Check sheet for the modelled part. Datum: model origin and axes. Units: mm. A direction names the side the tool comes from. Give positions to 0.01 mm unless a question says otherwise; leave off trailing zeros. Loops run counter-clockwise (first coordinate to the right, second up) from the corner with the lowest first, then second, coordinate; pieces in that order, holes last. Notation, with made-up numbers: (-22.5, 84.25) -> (3.5, 84.25) arc R30 cw to (3.5, 116.25) -> close; hole circle Ø9 at (-16.5, 51.5). An arc over 180 degrees is marked (long way). Answer as CSV lines item,"result". Start each with the question number.
(1) Material ranges on line 1 (Z direction, x = 36, y = -0.55); line 2 (X direction, y = -0.8, z = -69); line 3 (X direction, y = -18.15, z = -10), recorded low to high. Write a range as from..to.
(2) Section check B-B on x = -22.5. Enter the section's corners in (y, z), plus the area to 3 significant figures.
(3) Gauge pin test, flat ends, axial feed: pin 1 Ø3 at (x, z) = (36, -69) entering from +Y; pin 2 Ø3 at (x, z) = (-15.5, -29.5) entering from -Y; pin 3 Ø1.5 at (x, y) = (-18, -3) entering from -Z; pin 4 Ø1.5 at (x, z) = (-15.5, -10.5) entering from -Y. Record the tip position at first contact, or that the pin passes through.
(4) Access from +Z, -Z, +X, -X, +Y, -Y to the whole of each face (thin tool, end or side, straight path). Record for faces 1 (the face through (-40, 0, 0)), 2 (the face through (-24, -4, -66)), 3 (the face through (-18.31, -3.52, -18.97)).
(5) Section check C-C on y = -8.75. Enter the section's corners in (x, z).
(6) Section check A-A on x = 0. Enter the section's corners in (y, z).
(7) Section check D-D on z = -53.5. Enter the section's corners in (x, y).
(8) Release check for a two-part mould opening along X. For faces 4 (the face through (0, -1, 45)), 5 (the face through (-19, -3, -15)), 6 (the face through (40, 0, 0)), 7 (the face through (45, 0, -54)) record: pulls with the +X half, pulls with the -X half, needs draft (parallel to the pull), parting line crosses it, or undercut.
from build123d import *

# Parameters (mm, degrees)
SKETCH_1_W               = 100
SKETCH_1_H               = 150
EXTRUDE_2_DEPTH          = 2
SKETCH_3_R               = 1.75
CUT_EXTRUDE_1_DEPTH      = 91.227490268
MIRROR_2_COPY_1_SKETCH_R = 1.75
MIRROR_2_COPY_1_DEPTH    = 91.227490268
SKETCH_5_W               = 20
SKETCH_5_H               = 15
CUT_EXTRUDE_3_DEPTH      = 1
SKETCH_6_R               = 1.25
CUT_EXTRUDE_4_DEPTH      = 3
SKETCH_8_W               = 16
SKETCH_8_H               = 25
CUT_EXTRUDE_5_DEPTH      = 91.227490268
SKETCH_9_W               = 66
SKETCH_9_H               = 36
CUT_EXTRUDE_7_DEPTH      = 1
SKETCH_10_R              = 1.25
CUT_EXTRUDE_8_DEPTH      = 2
SKETCH_11_W              = 68
SKETCH_11_H              = 55
EXTRUDE_3_DEPTH          = 3
SKETCH_12_R              = 1.5
SKETCH_12_R_2            = 1.25
CUT_EXTRUDE_9_DEPTH      = 3
SKETCH_13_W              = 10
SKETCH_13_H              = 55
SKETCH_13_W_2            = 43
CUT_EXTRUDE_10_DEPTH     = 3
SKETCH_14_W              = 10
SKETCH_14_H              = 42
SKETCH_14_W_2            = 5
SKETCH_14_H_2            = 12.78
SKETCH_14_H_3            = 19.94
SKETCH_14_H_4            = 6.28
CUT_EXTRUDE_11_DEPTH     = 3
SKETCH_15_W              = 5
SKETCH_15_H              = 20.32
CUT_EXTRUDE_12_DEPTH     = 91.227490268
MIRROR_4_COPY_1_SKETCH_W = 5
MIRROR_4_COPY_1_SKETCH_H = 20.32
MIRROR_4_COPY_1_DEPTH    = 91.227490268
SKETCH_17_R              = 3
EXTRUDE_4_DEPTH          = 17
SKETCH_19_R              = 1.5
CUT_EXTRUDE_14_DEPTH     = 3
SKETCH_20_R              = 5
CUT_EXTRUDE_15_DEPTH     = 92.727858364


with BuildPart() as part:
    # 草图1 → 凸台-拉伸2 (new, symmetric)
    with BuildSketch(Plane(origin=(0, 0, 0), x_dir=(1, 0, 0), z_dir=(0, 1, 0))):
        Rectangle(SKETCH_1_W, SKETCH_1_H)
    extrude(amount=EXTRUDE_2_DEPTH, both=True)

    # 草图3 → 切除-拉伸1 (cut, through all)
    with BuildSketch(Plane(origin=(0, 2, 0), x_dir=(1, 0, 0), z_dir=(0, 1, 0))):
        with Locations(Location((-36, -19, 0), (0, 0, 270))):
            Circle(SKETCH_3_R)
        with Locations(Location((-36, -69, 0), (0, 0, 270))):
            Circle(SKETCH_3_R)
    cut_extrude_1 = extrude(amount=-CUT_EXTRUDE_1_DEPTH, mode=Mode.SUBTRACT)

    # 镜向1: 切除-拉伸1 across plane
    add(cut_extrude_1.mirror(Plane(origin=(0, 0, 0), x_dir=(0, 0, 1), z_dir=(1, 0, 0))), mode=Mode.SUBTRACT)

    # 镜向2: 切除-拉伸1 across plane
    add(cut_extrude_1.mirror(Plane.XY), mode=Mode.SUBTRACT)

    # 镜向2 copy 1 sketch → 镜向2 copy 1 (cut, through all)
    with BuildSketch(Plane(origin=(0, 2, 0), x_dir=(-1, 0, 0), z_dir=(0, 1, 0))):
        with Locations(Location((-36, -19, 0), (0, 0, 270))):
            Circle(MIRROR_2_COPY_1_SKETCH_R)
        with Locations(Location((-36, -69, 0), (0, 0, 270))):
            Circle(MIRROR_2_COPY_1_SKETCH_R)
    extrude(amount=-MIRROR_2_COPY_1_DEPTH, mode=Mode.SUBTRACT)

    # 草图5 → 切除-拉伸3 (cut)
    with BuildSketch(Plane.XZ.offset(2)):
        Rectangle(SKETCH_5_W, SKETCH_5_H)
    extrude(amount=-CUT_EXTRUDE_3_DEPTH, mode=Mode.SUBTRACT)

    # 草图6 → 切除-拉伸4 (cut)
    with BuildSketch(Plane.XZ.offset(1)):
        with Locations(Location((-8, 5.5, 0), (0, 0, 270))):
            Circle(SKETCH_6_R)
        with Locations(Location((8, 5.5, 0), (0, 0, 90))):
            Circle(SKETCH_6_R)
        with Locations(Location((8, -5.5, 0), (0, 0, 270))):
            Circle(SKETCH_6_R)
        with Locations(Location((-8, -5.5, 0), (0, 0, 90))):
            Circle(SKETCH_6_R)
    extrude(amount=-CUT_EXTRUDE_4_DEPTH, mode=Mode.SUBTRACT)

    # 草图8 → 切除-拉伸5 (cut, through all)
    with BuildSketch(Plane(origin=(0, 2, 0), x_dir=(1, 0, 0), z_dir=(0, 1, 0))):
        with Locations((-32, 0)):
            Rectangle(SKETCH_8_W, SKETCH_8_H)
        with Locations((32, 0)):
            Rectangle(SKETCH_8_W, SKETCH_8_H)
    extrude(amount=-CUT_EXTRUDE_5_DEPTH, mode=Mode.SUBTRACT)

    # 草图9 → 切除-拉伸7 (cut)
    with BuildSketch(Plane.XZ.offset(2)):
        with Locations((0, 45)):
            Rectangle(SKETCH_9_W, SKETCH_9_H)
    extrude(amount=-CUT_EXTRUDE_7_DEPTH, mode=Mode.SUBTRACT)

    # 草图10 → 切除-拉伸8 (cut)
    with BuildSketch(Plane.XZ.offset(1)):
        with Locations(Location((-30.48, 60.55, 0), (0, 0, 270))):
            Circle(SKETCH_10_R)
        with Locations(Location((30.48, 60.55, 0), (0, 0, 90))):
            Circle(SKETCH_10_R)
        with Locations(Location((30.48, 29.45, 0), (0, 0, 270))):
            Circle(SKETCH_10_R)
        with Locations(Location((-30.48, 29.45, 0), (0, 0, 90))):
            Circle(SKETCH_10_R)
    extrude(amount=-CUT_EXTRUDE_8_DEPTH, mode=Mode.SUBTRACT)

    # 草图11 → 凸台-拉伸3 (add)
    with BuildSketch(Plane.XZ.offset(2)):
        with Locations((0, -42.5)):
            Rectangle(SKETCH_11_W, SKETCH_11_H)
    extrude(amount=EXTRUDE_3_DEPTH)

    # 草图12 → 切除-拉伸9 (cut)
    with BuildSketch(Plane.XZ.offset(5)):
        with Locations(Location((-18.76, -17.54, 0), (0, 0, 270))):
            Circle(SKETCH_12_R)
        with Locations(Location((-18.76, -65.8, 0), (0, 0, 270))):
            Circle(SKETCH_12_R)
        with Locations(Location((32.04, -32.78, 0), (0, 0, 270))):
            Circle(SKETCH_12_R_2)
        with Locations(Location((32.04, -60.72, 0), (0, 0, 270))):
            Circle(SKETCH_12_R)
    extrude(amount=-CUT_EXTRUDE_9_DEPTH, mode=Mode.SUBTRACT)

    # 草图13 → 切除-拉伸10 (cut)
    with BuildSketch(Plane.XZ.offset(5)):
        with Locations((-29, -42.5)):
            Rectangle(SKETCH_13_W, SKETCH_13_H)
        with Locations((7.5, -42.5)):
            Rectangle(SKETCH_13_W_2, SKETCH_13_H)
    extrude(amount=-CUT_EXTRUDE_10_DEPTH, mode=Mode.SUBTRACT)

    # 草图14 → 切除-拉伸11 (cut)
    with BuildSketch(Plane.XZ.offset(5)):
        with Locations((-19, -41.742030173)):
            Rectangle(SKETCH_14_W, SKETCH_14_H)
        with Locations((31.5, -21.39)):
            Rectangle(SKETCH_14_W_2, SKETCH_14_H_2)
        with Locations((31.5, -47.75)):
            Rectangle(SKETCH_14_W_2, SKETCH_14_H_3)
        with Locations((31.5, -66.86)):
            Rectangle(SKETCH_14_W_2, SKETCH_14_H_4)
    extrude(amount=-CUT_EXTRUDE_11_DEPTH, mode=Mode.SUBTRACT)

    # 草图15 → 切除-拉伸12 (cut, through all)
    with BuildSketch(Plane.XZ.offset(2)):
        with Locations((-47.5, -54)):
            Rectangle(SKETCH_15_W, SKETCH_15_H)
    cut_extrude_12 = extrude(amount=-CUT_EXTRUDE_12_DEPTH, mode=Mode.SUBTRACT)

    # 镜向3: 切除-拉伸12 across plane
    add(cut_extrude_12.mirror(Plane.XY), mode=Mode.SUBTRACT)

    # 镜向4: 切除-拉伸12 across plane
    add(cut_extrude_12.mirror(Plane(origin=(0, 0, 0), x_dir=(0, 0, 1), z_dir=(1, 0, 0))), mode=Mode.SUBTRACT)

    # 镜向4 copy 1 sketch → 镜向4 copy 1 (cut, through all)
    with BuildSketch(Plane(origin=(0, -2, 0), x_dir=(-1, 0, 0), z_dir=(0, -1, 0))):
        with Locations((-47.5, -54)):
            Rectangle(MIRROR_4_COPY_1_SKETCH_W, MIRROR_4_COPY_1_SKETCH_H)
    extrude(amount=-MIRROR_4_COPY_1_DEPTH, mode=Mode.SUBTRACT)

    # 草图17 → 凸台-拉伸4 (add)
    with BuildSketch(Plane.XZ.offset(2)):
        with Locations(Location((15, 10, 0), (0, 0, 270))):
            Circle(SKETCH_17_R)
        with Locations(Location((-15, 10, 0), (0, 0, 90))):
            Circle(SKETCH_17_R)
        with Locations(Location((15, -10, 0), (0, 0, 90))):
            Circle(SKETCH_17_R)
        with Locations(Location((-15, -10, 0), (0, 0, 270))):
            Circle(SKETCH_17_R)
    extrude(amount=EXTRUDE_4_DEPTH)

    # 草图19 → 切除-拉伸14 (cut)
    with BuildSketch(Plane.XZ.offset(19)):
        with Locations(Location((15, 10, 0), (0, 0, 270))):
            Circle(SKETCH_19_R)
        with Locations(Location((-15, 10, 0), (0, 0, 90))):
            Circle(SKETCH_19_R)
        with Locations(Location((15, -10, 0), (0, 0, 90))):
            Circle(SKETCH_19_R)
        with Locations(Location((-15, -10, 0), (0, 0, 270))):
            Circle(SKETCH_19_R)
    extrude(amount=-CUT_EXTRUDE_14_DEPTH, mode=Mode.SUBTRACT)

    # 草图20 → 切除-拉伸15 (cut, through all)
    with BuildSketch(Plane.XZ.offset(2)):
        with Locations(Location((0, 18, 0), (0, 0, 270))):
            Circle(SKETCH_20_R)
        with Locations(Location((0, -18, 0), (0, 0, 90))):
            Circle(SKETCH_20_R)
    extrude(amount=-CUT_EXTRUDE_15_DEPTH, mode=Mode.SUBTRACT)


solid = part.part
Working result:
1,line 1,"z = -75..-70.75, -67.25..-20.75, -17.25..-12.5, 12.5..17.25, 20.75..67.25, 70.75..75"
1,line 2,"x = -50..-37.75, -34.25..34.25, 37.75..50"
1,line 3,"x = -18..-16.5, -13.5..-12, 12..13.5, 16.5..18"
2,outline,"(-5, -70) -> (-2, -70) -> (-2, -75) -> (2, -75) -> (2, 75) -> (-2, 75) -> (-2, 63) -> (-1, 63) -> (-1, 27) -> (-2, 27) -> (-2, -15) -> (-5, -15) -> (-5, -20.74) -> (-2, -20.74) -> (-2, -62.74) -> (-5, -62.74) -> close"
2,area,"603 mm^2"
3,pin 1,"passes through"
3,pin 2,"stops at y = -2"
3,pin 3,"stops at z = -70"
3,pin 4,"stops at y = -16"
4,face 1,"+Y, -Y"
4,face 2,"+Z, -Z, -X, -Y"
4,face 3,"-Y"
5,outline,"circle Ø6 at (-15, -10); circle Ø6 at (-15, 10); circle Ø6 at (15, -10); circle Ø6 at (15, 10)"
6,outline,"(-2, -75) -> (2, -75) -> (2, -23) -> (-2, -23) -> close; (-2, -13) -> (2, -13) -> (2, 13) -> (-2, 13) -> (-2, 7.5) -> (-1, 7.5) -> (-1, -7.5) -> (-2, -7.5) -> close; (-2, 23) -> (2, 23) -> (2, 75) -> (-2, 75) -> (-2, 63) -> (-1, 63) -> (-1, 27) -> (-2, 27) -> close"
7,outline,"(-45, -2) -> (45, -2) -> (45, 2) -> (-45, 2) -> close"
8,face 4,"undercut"
8,face 5,"needs draft"
8,face 6,"undercut"
8,face 7,"pulls with the +X half"
